Here's how the part is built. I have some questions about the finished solid (model axes, mm). Face numbers are marked on the shaded views. A direction names the side the tool comes from. Give positions to 0.01 mm unless a question says otherwise; leave off trailing zeros. Write each loop counter-clockwise with the first axis right and the second up, starting at its lowest first coordinate (ties: lowest second). Pieces come first, ordered by that corner, then holes. Notation, with made-up numbers: (29.5, -40) -> (51.5, -40) arc R24 cw to (51.5, -5) -> close; hole circle Ø1 at (-35.75, 35). An arc over 180 degrees is marked (long way). Answer as CSV lines item,"result". Start each with the question number.
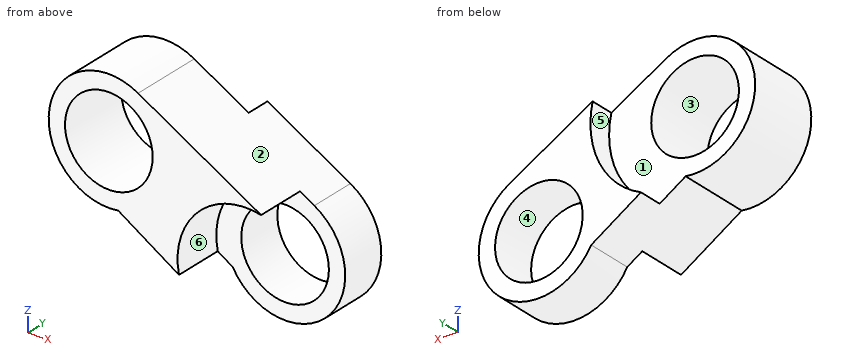
from build123d import *

# Parameters (mm, degrees)
SKETCH012_R       = 2.55
PAD010_DEPTH      = 5.6
CYLINDER008_R     = 5
CYLINDER008_DEPTH = 10
CYLINDER009_R     = 4
CYLINDER009_DEPTH = 8


with BuildPart() as part:
    # Sketch012 → Pad010 (new body)
    with BuildSketch(Plane.XZ.offset(6.2)):
        with BuildLine():
            ThreePointArc((4.954527, 54.655154), (10.483926, 53.914212), (9.702481, 59.438032))
            Line((1.702481, 63.891826), (9.702481, 59.438032))
            ThreePointArc((1.702481, 63.891826), (-3.446315, 61.444457), (0.548094, 57.376976))
            Line((0.548094, 57.376976), (4.954527, 54.655154))
        make_face()
        with Locations((8, 56.38)):
            Circle(SKETCH012_R, mode=Mode.SUBTRACT)
        with Locations((0, 60.833794)):
            Circle(SKETCH012_R, mode=Mode.SUBTRACT)
    extrude(amount=PAD010_DEPTH)

    # Cylinder008 → Cylinder008 (cut)
    with BuildSketch(Plane(origin=(0, 2.4, 61), x_dir=(1, 0, 0), z_dir=(0, -1, 0))):
        Circle(CYLINDER008_R)
    extrude(amount=CYLINDER008_DEPTH, mode=Mode.SUBTRACT)

    # Cylinder009 → Cylinder009 (cut)
    with BuildSketch(Plane(origin=(8, -8.9, 56), x_dir=(1, 0, 0), z_dir=(0, -1, 0))):
        Circle(CYLINDER009_R)
    extrude(amount=CYLINDER009_DEPTH, mode=Mode.SUBTRACT)


solid = part.part
Item 1: If we section it at C-C (x = 8): Please give me the cut outline in (y, z).
Item 2: If we section it at B-B (z = 62.75): Please give me the cut outline in (x, y).
Item 3: For the marked faces 4, 5 and 6, which set-ups out of +Z, -Z, +X, -X, +Y, -Y let a thin tool reach every point of the face, with its end or its side?
Item 4: If I drill on line 1 (Z direction, x = 0, y = -9.4); line 2 (Y direction, x = 2, z = 58); line 3 (X direction, y = -10.95, z = 60.75), over which ranges is the centre line in solid material (lowest first)? Write a range as [from, to].
Item 5: I'm going to push flat-ended pins straight in: pin 1 (1 mm diameter, centred on x = 4.5, y = -11, fed in from -Z); pin 2 (1.5 mm diameter, centred on x = 4.5, y = -10.5, fed in from +Z); pin 3 (3 mm diameter, centred on y = -9, z = 54.5, fed in from +X). Where does each tip first touch, or does it pass through?
Item 6: We'd pull the mould along X, two halves only. Please class the marked faces 1, 2 and 3: released by +X, released by -X, zero draft, split by the parting line, or undercut.
Item 7: If we section it at D-D (y = -9.3): Please give me the cut outline in (x, z), and give its area (3 significant figures).
Item 8: If we section it at A-A (x = 0): Please give me the cut outline in (y, z).
Final values:
1,outline,"(-11.8, 60) -> (-8.9, 60) -> (-8.9, 58.93) -> (-6.2, 58.93) -> (-6.2, 60.39) -> (-11.8, 60.39) -> close; (-8.9, 52.88) -> (-6.2, 52.88) -> (-6.2, 53.83) -> (-8.9, 53.83) -> close"
2,outline,"(-2.93, -11.8) -> (-1.68, -11.8) -> (-1.68, -7.6) -> (-2.93, -7.6) -> close; (1.68, -11.8) -> (3.75, -11.8) -> (3.75, -7.6) -> (1.68, -7.6) -> close"
3,face 4,"+Y, -Y"
3,face 5,"-X, +Y"
3,face 6,"-Y"
4,line 1,"[57.33, 58.28], [63.38, 64.33]"
4,line 2,"[-11.8, -7.6]"
4,line 3,"[-3.5, -2.55], [2.55, 7.35]"
5,pin 1,"z = 55.19"
5,pin 2,"z = 62.75"
5,pin 3,"x = 11.48"
6,face 1,"zero draft"
6,face 2,"released by +X"
6,face 3,"undercut"
7,outline,"(0.55, 57.38) -> (4.08, 55.19) arc R4 cw to (8.86, 59.91) -> (1.7, 63.89) arc R3.5 ccw (long way) to start; hole circle Ø5.1 at (0, 60.83)"
7,area,"37.2 mm2"
8,outline,"(-11.8, 57.33) -> (-7.6, 57.33) -> (-7.6, 58.28) -> (-11.8, 58.28) -> close; (-11.8, 63.38) -> (-7.6, 63.38) -> (-7.6, 64.33) -> (-11.8, 64.33) -> close"
